from build123d import *

# Parameters (mm, degrees)
BOSS_EXTRUDE1_DEPTH = 127
SKETCH2_R           = 6.35
BOSS_EXTRUDE3_DEPTH = 44.45


with BuildPart() as part:
    # Sketch1 → Boss-Extrude1 (new body)
    with BuildSketch(Plane(origin=(0, 0, 0), x_dir=(1, 0, 0), z_dir=(0, 1, 0))):
        with BuildLine():
            ThreePointArc((25.626778658, -38.1), (18.122521252, -20.031067918), (0, -12.657167374))
            ThreePointArc((0, -12.657167374), (-18.122521252, -20.031067918), (-25.626778658, -38.1))
            Line((-25.626778658, -38.1), (-25.626778658, -57.15))
            Line((-25.626778658, -57.15), (-44.676778658, -57.15))
            Line((-44.676778658, -57.15), (-44.676778658, -19.05))
            Line((-44.676778658, -19.05), (-22.225, 0))
            Line((-22.225, 0), (22.225, 0))
            Line((22.225, 0), (44.676778658, -19.05))
            Line((44.676778658, -19.05), (44.676778658, -57.15))
            Line((44.676778658, -57.15), (25.626778658, -57.15))
            Line((25.626778658, -57.15), (25.626778658, -38.1))
        make_face()
    extrude(amount=-BOSS_EXTRUDE1_DEPTH)

    # Sketch2 → Boss-Extrude3 (add)
    with BuildSketch(Plane(origin=(-22.225, 0, 0), x_dir=(0, 1, 0), z_dir=(-1, 0, 0))):
        with BuildLine():
            Line((-127, 0), (-127, 31.75))
            ThreePointArc((-127, 31.75), (-114.3, 44.45), (-101.6, 31.75))
            Line((-101.6, 31.75), (-101.6, 20.00617362))
            Line((-101.6, 20.00617362), (-25.4, 20.00617362))
            Line((-25.4, 20.00617362), (-25.4, 31.75))
            Line((-25.4, 31.75), (0, 31.75))
            Line((0, 31.75), (0, 0))
            Line((0, 0), (-127, 0))
        make_face()
        with Locations(Location((-114.3, 31.75, 0), (0, 0, 270))):
            Circle(SKETCH2_R, mode=Mode.SUBTRACT)
    extrude(amount=-BOSS_EXTRUDE3_DEPTH)


solid = part.part
Geometry check sheet. Reference: the model listing, model coordinates, mm. A direction names the side the tool comes from. Give positions to 0.01 mm unless a question says otherwise; leave off trailing zeros. Order: outer loops, then holes, each group sorted by start corner. A loop starts at its lowest first (then second) coordinate and runs counter-clockwise, first axis right, second up. Notation, with made-up numbers: M -18.75,-12.5 L 3.25,-12.5 A23 ccw 3.25,11.5 Z; hole C 56,39.5 d11. An arc over 180 degrees is marked long. Use a Markdown table: item, result.
Item 1: Draft check along X on faces 1 (the flat face through (-25.627, -63, 47)), 2 (the flat face through (-33.61, -62.61, 9.66)), 3 (the cylindrical face through (-0.311, -108.946, -28.336)). Enter one of: +X half, -X half, draft (parallel to the pull), parting line (faces both ways), or undercut.
Answers follow:
| item | result |
|---|---|
| face 1 | undercut |
| face 2 | -X half |
| face 3 | draft |
Item 2: Section check C-C (y = -114.3). Record the cut outline in (x, z) (3 decimals), and give its area (3 significant figures).
Answers follow:
| item | result |
|---|---|
| outline | M -44.677,19.05 L -22.225,0 L -22.225,-25.4 L 22.225,-25.4 L 22.225,0 L 44.677,19.05 L 44.677,57.15 L 25.627,57.15 L 25.627,38.1 A25.4 cw 0,12.657 A25.4 cw -25.627,38.1 L -25.627,57.15 L -44.677,57.15 Z; M -22.225,-44.45 L 22.225,-44.45 L 22.225,-38.1 L -22.225,-38.1 Z |
| area | 4,090 mm2 |
Item 3: Tool access check on faces 4 (the flat face through (0, -64, -20.006)), 5 (the flat face through (25.627, -63, 48)), 6 (the flat face through (-22.225, -63, -13)), 7 (the flat face through (22.225, -63, -13)). Record the directions out of +Z, -Z, +X, -X, +Y, -Y that give a thin tool (end or side, any length) a straight path to the whole face; none if there is none.
Answers follow:
| item | result |
|---|---|
| face 4 | -Z, +X, -X |
| face 5 | +Z, +Y, -Y |
| face 6 | -Z, -X, +Y, -Y |
| face 7 | -Z, +X, +Y, -Y |
Item 4: Section check D-D (z = 10.5). Record the cut outline in (x, y), and give its area (3 significant figures).
Answers follow:
| item | result |
|---|---|
| outline | M -34.6,-127 L 34.6,-127 L 34.6,0 L -34.6,0 Z |
| area | 8,790 mm2 |
Item 5: Section check B-B (x = -2.5). Record the cut outline in (y, z), and give its area (3 significant figures).
Answers follow:
| item | result |
|---|---|
| outline | M -127,-31.75 A12.7 ccw -101.6,-31.75 L -101.6,-20.01 L -25.4,-20.01 L -25.4,-31.75 L 0,-31.75 L 0,12.76 L -127,12.76 Z; hole C -114.3,-31.75 d12.7 |
| area | 4,880 mm2 |
Item 6: Material ranges on line 1 along X through (y, z) = (-88.5, 43); line 2 along X through (y, z) = (-20.5, -10.5) (3 decimals); line 3 along Y through (x, z) = (-10, -31), recorded low to high.
Answers follow:
| item | result |
|---|---|
| line 1 | x = -44.68 to -25.63, 25.63 to 44.68 |
| line 2 | x = -22.225 to 22.225 |
| line 3 | y = -127 to -120.61, -107.99 to -101.6, -25.4 to 0 |
Item 7: Depth check by flat-ended pin: P1, Ø10, axis at x = 19, y = -75.5, coming from the -Z side; P2, Ø1, axis at y = -50, z = -21, coming from the +X side (1 decimal); P3, Ø22, axis at y = -68.5, z = -17, coming from the -X side (3 decimals); P4, Ø20.5, axis at y = -114.3, z = -31.75, coming from the +X side (3 decimals). Enter the tip coordinate at first touch or a pass-through.
Answers follow:
| item | result |
|---|---|
| P1 | stops at z = -20.01 |
| P2 | passes through |
| P3 | stops at x = -22.225 |
| P4 | stops at x = 22.225 |
Item 8: Section check A-A (z = 43). Record the cut outline in (x, y).
Answers follow:
| item | result |
|---|---|
| outline | M -44.68,-127 L -25.63,-127 L -25.63,0 L -44.68,0 Z; M 25.63,-127 L 44.68,-127 L 44.68,0 L 25.63,0 Z |
